Autodesk Fusion 360 part; units mm, degrees
sketch "Sketch1" plane through (0, 0, 0) normal (0, 1, 0) x (1, 0, 0)
sketch "Sketch2" plane through (0, 0, 0) normal (0, 0, 1) x (1, 0, 0)
  line L0 (50, 0) -> (50, -40)
  line L1 (50, -40) -> (-50, -40)
  line L2 (-50, -40) -> (-50, 40)
  line L3 (-50, 40) -> (50, 40)
  line L4 (50, 40) -> (50, -40)
extrude "Extrude1" add sketch "Sketch2" along normal blind 10
sketch "Sketch3" plane through (0, 0, 10) normal (0, 0, 1) x (-1, 0, 0)
  line L0 (-50, -40) -> (50, -40)
  line L1 (50, -40) -> (50, 40)
  line L2 (50, 40) -> (-50, 40)
  line L3 (-50, 40) -> (-50, -40)
  line L4 (50, 40) -> (15, 40)
  line L5 (15, 40) -> (15, 32)
  line L6 (15, 32) -> (42, 32)
  line L7 (42, 32) -> (42, 5)
  line L8 (42, 5) -> (50, 5)
  line L9 (50, 5) -> (50, 40)
  dimension "d6" = 35
  dimension "d9" = 35
extrude "Extrude2" add sketch "Sketch3" along normal blind 15 contours L1 L2 L4 L5 L6 L7 L8 L9
sketch "Sketch4" plane through (0, 0, 10) normal (0, 0, 1) x (-1, 0, 0)
  line L0 (15, 32) -> (15, 40)
  line L1 (15, 40) -> (-50, 40)
  line L2 (-50, 40) -> (-50, -40)
  line L3 (-50, -40) -> (50, -40)
  line L4 (50, -40) -> (50, 5)
  line L5 (50, 5) -> (42, 5)
  line L6 (42, 5) -> (42, 32)
  line L7 (42, 32) -> (15, 32)
  line L8 (15, 32) -> (-15, 32)
  line L9 (-15, 32) -> (-15, 40)
  line L10 (-15, 40) -> (15, 40)
  line L11 (15, 40) -> (15, 32)
  dimension "d12" = 30
extrude "Extrude3" add sketch "Sketch4" along normal blind 7 contours L0 L1 L8 L9 L10 L11
sketch "Sketch5" plane through (0, 0, 10) normal (0, 0, 1) x (-1, 0, 0)
  line L0 (-15, 32) -> (-15, 40)
  line L1 (-15, 40) -> (-50, 40)
  line L2 (-50, 40) -> (-50, -40)
  line L3 (-50, -40) -> (50, -40)
  line L4 (50, -40) -> (50, 5)
  line L5 (50, 5) -> (42, 5)
  line L6 (42, 5) -> (42, 32)
  line L7 (42, 32) -> (-15, 32)
  line L8 (-15, 32) -> (-42, 32)
  line L9 (-50, 40) -> (-15, 40)
  line L10 (-15, 40) -> (-15, 32)
  line L11 (-42, 32) -> (-42, 12)
  line L12 (-42, 12) -> (-50, 12)
  line L13 (-50, 12) -> (-50, 40)
  dimension "d16" = 28
extrude "Extrude4" add sketch "Sketch5" along normal blind 15 contours L0 L1 L2 L8 L9 L10 L11 L12 L13
sketch "Sketch6" plane through (0, 0, 10) normal (0, 0, 1) x (-1, 0, 0)
  line L0 (-42, 12) -> (-50, 12)
  line L1 (-50, 12) -> (-50, -40)
  line L2 (-50, -40) -> (50, -40)
  line L3 (50, -40) -> (50, 5)
  line L4 (50, 5) -> (42, 5)
  line L5 (42, 5) -> (42, 32)
  line L6 (42, 32) -> (-42, 32)
  line L7 (-42, 32) -> (-42, 12)
  line L8 (42, -32) -> (42, -5)
  line L9 (42, -5) -> (50, -5)
  line L10 (50, -5) -> (50, -40)
  line L11 (50, -40) -> (15, -40)
  line L12 (15, -40) -> (15, -32)
  line L13 (15, -32) -> (42, -32)
  dimension "d19" = 35
  dimension "d20" = 35
sketch "Sketch7" plane through (0, 0, 10) normal (0, 0, 1) x (-1, 0, 0)
  line L0 (-50, -40) -> (-42, -40)
  line L1 (-42, -32) -> (-42, -12)
  line L2 (-42, -12) -> (-50, -12)
  line L3 (-50, -12) -> (-50, -40)
  line L4 (-50, -40) -> (-15, -40)
  line L5 (-15, -40) -> (-15, -32)
  line L6 (-15, -32) -> (-42, -32)
  line L7 (-50, -32) -> (-50, -40)
  dimension "d22" = 8
  dimension "d23" = 28
  dimension "d24" = 35
  dimension "d25" = 8
extrude "Extrude5" add sketch "Sketch7" sketch "Sketch6" along normal blind 15 of sketch 2 contours L2 L3 L8 L9 L10 L11 L12 L13
sketch "Sketch8" plane through (0, 0, 10) normal (0, 0, 1) x (-1, 0, 0)
  line L0 (42, -5) -> (50, -5)
  line L1 (50, -5) -> (50, 5)
  line L2 (50, 5) -> (42, 5)
  line L3 (42, 5) -> (42, 32)
  line L4 (42, 32) -> (-42, 32)
  line L5 (-42, 32) -> (-42, 12)
  line L6 (-42, 12) -> (-50, 12)
  line L7 (-50, 12) -> (-50, -12)
  line L8 (-50, -12) -> (-42, -12)
  line L9 (-42, -12) -> (-42, -32)
  line L10 (-42, -32) -> (-15, -32)
  line L11 (-15, -32) -> (-15, -40)
  line L12 (-15, -40) -> (15, -40)
  line L13 (15, -40) -> (15, -32)
  line L14 (15, -32) -> (42, -32)
  line L15 (42, -32) -> (42, -5)
sketch "Sketch9" plane through (0, 0, 25) normal (0, 0, 1) x (-1, 0, 0)
  line L0 (-50, 12) -> (-42, 12)
  line L1 (-42, 12) -> (-42, 32)
  line L2 (-42, 32) -> (-15, 32)
  line L3 (-15, 32) -> (-15, 40)
  line L4 (-15, 40) -> (-50, 40)
  line L5 (-50, 40) -> (-50, 12)
sketch "Sketch10" plane through (0, 0, 10) normal (0, 0, 1) x (-1, 0, 0)
  line L0 (-50, 12) -> (-42, 12)
  line L1 (-42, 12) -> (-42, -12)
  line L2 (-42, -12) -> (-50, -12)
  line L3 (-50, -12) -> (-50, 12)
extrude "Extrude6" add sketch "Sketch10" along normal blind 35
sketch "Sketch11" plane through (0, 0, 10) normal (0, 0, 1) x (-1, 0, 0)
sketch "Sketch12" plane through (50, 0, 0) normal (1, 0, 0) x (0, 1, 0)
  line L0 (-40, 0) -> (40, 0)
  line L1 (40, 0) -> (40, 25)
  line L2 (40, 25) -> (12, 25)
  line L3 (12, 25) -> (12, 45)
  line L4 (12, 45) -> (-12, 45)
  line L5 (-12, 45) -> (-12, 25)
  line L6 (-12, 25) -> (-40, 25)
  line L7 (-40, 25) -> (-40, 0)
ref_plane "WorkPlane1" through (50, -12, 45) normal (1, 0, 0) x (0, 1, 0)
sketch "Sketch13" plane through (50, 0, 0) normal (1, 0, 0) x (0, 1, 0)
  line L0 (0, 37) -> (5, 37)
  line L1 (5, 37) -> (-5, 37)
  line L2 (-5, 37) -> (-5, 10)
  line L3 (-5, 10) -> (5, 10)
  line L4 (5, 10) -> (5, 37)
  dimension "d31" = 5
  dimension "d32" = 27
extrude "Extrude7" cut sketch "Sketch13" against normal blind 200
sketch "Sketch14" plane through (0, 0, 10) normal (0, 0, 1) x (-1, 0, 0)
  line L0 (-20, 0) -> (-20, 7.5)
  line L1 (20, 0) -> (20, -7.5)
  line L2 (-20, -7.5) -> (-20, 0)
  line L3 (10, -7.5) -> (10, -12.5)
  line L4 (10, -12.5) -> (-10, -12.5)
  line L5 (-10, -12.5) -> (-10, -7.5)
  line L6 (20, -7.5) -> (10, -7.5)
  line L7 (-10, -7.5) -> (-20, -7.5)
  line L8 (10, 12.5) -> (-10, 12.5)
  line L9 (10, 7.5) -> (10, 12.5)
  line L10 (20, 7.5) -> (10, 7.5)
  line L11 (20, 0) -> (20, 7.5)
  line L12 (-10, 12.5) -> (-10, 7.5)
  line L13 (-10, 7.5) -> (-20, 7.5)
  line L14 (-20, 7.5) -> (-20, 0)
  dimension "d35" = 20
  dimension "d36" = 7.5
  dimension "d37" = 15
  dimension "d40" = 20
  dimension "d41" = 5
extrude "Extrude8" cut sketch "Sketch14" against normal blind 100
sketch "Sketch15" plane through (0, -40, 0) normal (0, -1, 0) x (1, 0, 0)
  line L0 (-50, 0) -> (50, 0)
  line L1 (50, 0) -> (50, 25)
  line L2 (50, 25) -> (15, 25)
  line L3 (15, 25) -> (15, 17)
  line L4 (15, 17) -> (-15, 17)
  line L5 (-15, 17) -> (-15, 25)
  line L6 (-15, 25) -> (-50, 25)
  line L7 (-50, 25) -> (-50, 0)
sketch "Sketch16" plane through (0, 0, 10) normal (0, 0, 1) x (-1, 0, 0)
sketch "Sketch17" plane through (0, 0, 10) normal (0, 0, 1) x (-1, 0, 0)
  line L0 (-15, -32) -> (15, -32)
  line L1 (15, -32) -> (15, -40)
  line L2 (15, -40) -> (-15, -40)
  line L3 (-15, -40) -> (-15, -32)
extrude "Extrude9" add sketch "Sketch17" along normal blind 7
Geometry check sheet. Reference: the model listing, model coordinates, mm. A direction names the side the tool comes from. Give positions to 0.01 mm unless a question says otherwise; leave off trailing zeros. Loops run counter-clockwise (first coordinate to the right, second up) from the corner with the lowest first, then second, coordinate; pieces in that order, holes last. Notation, with made-up numbers: (89, 83.5) - (122, 83.5) arc R28 cw to (122, 110.5) - close; hole circle Ø2 at (62.25, 38). An arc over 180 degrees is marked (long way). Use CSV: the item, a comma, the result in double quotes. Start each with the question number.
Q1. Go/stop test with flat-tipped pins: pin 1 Ø6.5 at (x, y) = (-4.5, 35.5) entering from +Z; pin 2 Ø6 at (x, y) = (25, 28) entering from +Z; pin 3 Ø12 at (y, z) = (-15.5, 32.5) entering from -X. Record where each tip stops, or that it passes through.
Q2. Release check for a two-part mould opening along X. For faces 5 (the face through (-20, 0, 5)), 6 (the face through (-1, 40, 12)) record: +X half, -X half, draft (parallel to the pull), parting line (faces both ways), or undercut.
Q3. Section check B-B, the plane y = -0.5. Record the cut outline in (x, z), and give its area (3 significant figures).
Q4. Section check C-C, the plane z = 5.5. Record the cut outline in (x, y), and give its area (3 significant figures).
Q5. Access from +Z, -Z, +X, -X, +Y, -Y to the whole of each face (thin tool, end or side, straight path). Record for faces 1 (the face through (-40, 34, 25)), 2 (the face through (-42, -19, 17)), 3 (the face through (46, 0, 37)), 4 (the face through (-15, 7.5, 5)).
Q6. Section check D-D, the plane x = -6.5. Record the cut outline in (y, z), and give its area (3 significant figures).
Q7. Scan lines: probe 1 along Y at (x, z) = (36, 12); probe 2 along X at (y, z) = (-5, 3.5); probe 3 along X at (y, z) = (20, 12.5). Record each from-to range of solid material in increasing order. Write a range as from..to.
Q8. Section check A-A, the plane z = 12. Record the cut outline in (x, y).
Findings below:
1,pin 1,"stops at z = 17"
1,pin 2,"stops at z = 10"
1,pin 3,"stops at x = 42"
2,face 5,"undercut"
2,face 6,"draft"
3,outline,"(-50, 0) - (-20, 0) - (-20, 10) - (-50, 10) - close; (20, 0) - (50, 0) - (50, 10) - (20, 10) - close; (42, 37) - (50, 37) - (50, 45) - (42, 45) - close"
3,area,"664 mm^2"
4,outline,"(-50, -40) - (50, -40) - (50, 40) - (-50, 40) - close; hole (-20, -7.5) - (-10, -7.5) - (-10, -12.5) - (10, -12.5) - (10, -7.5) - (20, -7.5) - (20, 7.5) - (10, 7.5) - (10, 12.5) - (-10, 12.5) - (-10, 7.5) - (-20, 7.5) - close"
4,area,"7,200 mm^2"
5,face 1,"+Z, -X, +Y, -Y"
5,face 2,"+Z"
5,face 3,"+X, -X"
5,face 4,"+Z, -Z"
6,outline,"(-40, 0) - (-12.5, 0) - (-12.5, 10) - (-32, 10) - (-32, 17) - (-40, 17) - close; (12.5, 0) - (40, 0) - (40, 17) - (32, 17) - (32, 10) - (12.5, 10) - close"
6,area,"662 mm^2"
7,probe 1,"y = -40..-32, 32..40"
7,probe 2,"x = -50..-20, 20..50"
7,probe 3,"x = -50..-42, 42..50"
8,outline,"(-50, -40) - (50, -40) - (50, -5) - (42, -5) - (42, -32) - (-42, -32) - (-42, -5) - (-50, -5) - close; (-50, 5) - (-42, 5) - (-42, 32) - (42, 32) - (42, 5) - (50, 5) - (50, 40) - (-50, 40) - close"
